Source: CAD feature listing. Evaluate the final solid. Frame: model axes, mm. A direction names the side the tool comes from. Round coordinates to 2 decimals unless told otherwise and drop trailing zeros. Loops run counter-clockwise (first coordinate to the right, second up) from the corner with the lowest first, then second, coordinate; pieces in that order, holes last. Notation, with made-up numbers: (7.25, 41.25) -> (35.25, 41.25) arc R25 cw to (35.25, 73.25) -> close; hole circle Ø2 at (77, 19). An arc over 180 degrees is marked (long way). Put each result on its own line as item: value. Start each with the question number.
1. Contact query for flat-ended pins moving along their axis: pin 1 (3 mm diameter, centred on y = 13.5, z = -3.5, fed in from -X); pin 2 (3 mm diameter, centred on y = 11, z = -2, fed in from -X); pin 3 (5 mm diameter, centred on y = 4.5, z = 3, fed in from -X). Output: stop coordinate, or through.
2. Cut plane B-B (z = 0). Return the cut outline in (x, y) (3 decimals), then the cut area to 3 significant figures.
3. Material intervals for L1, parallel to Z at x = 81, y = 10.5 (3 decimals); L2, parallel to X at y = 14, z = -3; L3, parallel to Z at x = 112, y = 17.5, sorted ascending.
4. Cut plane A-A (x = -167). Return the cut outline in (y, z), then the cut area to 3 significant figures.
5. Set-up query: faces 5 (the flat face through (-26, 9.525, 0)), 6 (the flat face through (3, 9, -31.75)), 7 (the flat face through (-181, 10, 4.064)). Return all of +Z, -Z, +X, -X, +Y, -Y with unobstructed straight access to the full face (end or side cutting, diameter ignored); none if empty.
6. Draft query along X for faces 1 (the flat face through (-3, 0, 0)), 2 (the flat face through (228.6, 9, 0)), 3 (the flat face through (127, 10, 4.064)), 4 (the flat face through (-26, 14, -9.525)). Return one class per face: pulls with the +X half, pulls with the -X half, needs draft (parallel to the pull), parting line crosses it, or undercut.
7. Cut plane C-C (x = -62). Return the cut outline in (y, z) (3 decimals), then the cut area to 3 significant figures.
```python
from build123d import *

# Parameters (mm, degrees)
SKETCH1_W           = 457.2
SKETCH1_H           = 63.5
BOSS_EXTRUDE1_DEPTH = 19.05
CUT_EXTRUDE1_DEPTH  = 19.05
CUT_EXTRUDE2_DEPTH  = 232.579198116
SKETCH5_W           = 241.3
SKETCH5_H           = 19.05
CUT_EXTRUDE3_DEPTH  = 9.525


with BuildPart() as part:
    # Sketch1 → Boss-Extrude1 (new body)
    with BuildSketch(Plane(origin=(0, 0, 0), x_dir=(1, 0, 0), z_dir=(0, 1, 0))):
        Rectangle(SKETCH1_W, SKETCH1_H)
    extrude(amount=BOSS_EXTRUDE1_DEPTH)

    # Sketch2 → Cut-Extrude1 (cut)
    with BuildSketch(Plane(origin=(0, 19.05, 0), x_dir=(1, 0, 0), z_dir=(0, 1, 0))):
        with BuildLine():
            Line((146.05, -4.064), (107.95, -4.064))
            ThreePointArc((107.95, -4.064), (103.886, 0), (107.95, 4.064))
            Line((107.95, 4.064), (146.05, 4.064))
            ThreePointArc((146.05, 4.064), (150.114, 0), (146.05, -4.064))
        make_face()
        with BuildLine():
            Line((-200.025, 4.064), (-161.925, 4.064))
            ThreePointArc((-161.925, 4.064), (-157.861, 0), (-161.925, -4.064))
            Line((-161.925, -4.064), (-200.025, -4.064))
            ThreePointArc((-200.025, -4.064), (-204.089, 0), (-200.025, 4.064))
        make_face()
    extrude(amount=-CUT_EXTRUDE1_DEPTH, mode=Mode.SUBTRACT)

    # Sketch3 → Cut-Extrude2 (cut, through all)
    with BuildSketch(Plane(origin=(0, 19.05, 0), x_dir=(1, 0, 0), z_dir=(0, 1, 0))):
        Polygon((-228.6, 31.75), (-228.6, -31.75), (-215.9, 31.75), align=None)
    extrude(amount=-CUT_EXTRUDE2_DEPTH, mode=Mode.SUBTRACT)

    # Sketch5 → Cut-Extrude3 (cut)
    with BuildSketch(Plane(origin=(0, 19.05, 0), x_dir=(1, 0, 0), z_dir=(0, 1, 0))):
        with Locations((-24.511, 0)):
            Rectangle(SKETCH5_W, SKETCH5_H)
    extrude(amount=-CUT_EXTRUDE3_DEPTH, mode=Mode.SUBTRACT)


solid = part.part
```
Solution:
1. pin 1: stops at x = -221.85
1. pin 2: stops at x = -222.15
1. pin 3: stops at x = -223.35
2. outline: (-222.25, 0) -> (-204.089, 0) -> (-204.089, 19.05) -> (-222.25, 19.05) -> close; (-157.861, 0) -> (103.886, 0) -> (103.886, 19.05) -> (96.139, 19.05) -> (96.139, 9.525) -> (-145.161, 9.525) -> (-145.161, 19.05) -> (-157.861, 19.05) -> close; (150.114, 0) -> (228.6, 0) -> (228.6, 19.05) -> (150.114, 19.05) -> close
2. area: 4,530 mm^2
3. L1: z = -31.75 to -9.525, 9.525 to 31.75
3. L2: x = -221.65 to -202.77, -159.18 to -145.16, 96.14 to 105.21, 148.79 to 228.6
3. L3: z = -31.75 to -4.06, 4.06 to 31.75
4. outline: (0, -31.75) -> (19.05, -31.75) -> (19.05, -4.06) -> (0, -4.06) -> close; (0, 4.06) -> (19.05, 4.06) -> (19.05, 31.75) -> (0, 31.75) -> close
4. area: 1,050 mm^2
5. face 5: +Y
5. face 6: -Z, +X, -X, +Y, -Y
5. face 7: +Y, -Y
6. face 1: needs draft
6. face 2: pulls with the +X half
6. face 3: undercut
6. face 4: undercut
7. outline: (0, -31.75) -> (19.05, -31.75) -> (19.05, -9.525) -> (9.525, -9.525) -> (9.525, 9.525) -> (19.05, 9.525) -> (19.05, 31.75) -> (0, 31.75) -> close
7. area: 1,030 mm^2
